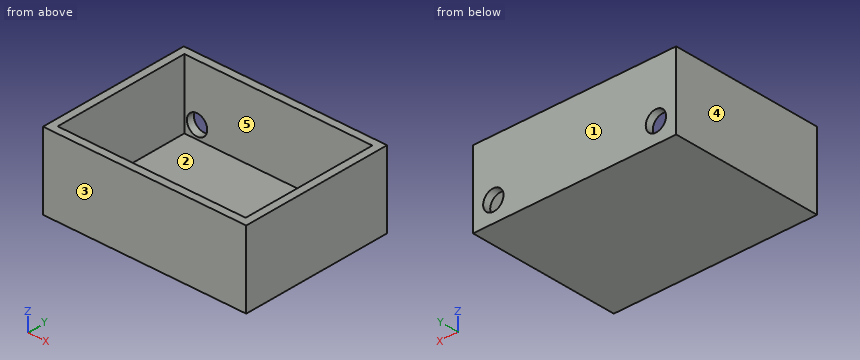
from build123d import *

# Parameters (mm, degrees)
F0_W     = 74
F0_H     = 54
F1_DEPTH = 3
F0_W_2   = 80
F0_H_2   = 60
F2_DEPTH = 30
F3_R     = 4
F4_DEPTH = 5


with BuildPart() as f1:
    # F0 (on Top) → F1 (new body)
    with BuildSketch(Plane.XY):
        with Locations((40, -30)):
            Rectangle(F0_W, F0_H)
    extrude(amount=F1_DEPTH)

    # F0 (on Top) → F2 (join)
    with BuildSketch(Plane.XY):
        with Locations((40, -30)):
            Rectangle(F0_W_2, F0_H_2)
        with Locations((40, -30)):
            Rectangle(F0_W, F0_H, mode=Mode.SUBTRACT)
    extrude(amount=F2_DEPTH)

    # F3 (on Front) → F4 (cut)
    with BuildSketch(Plane.XZ):
        with Locations((72, 8)):
            Circle(F3_R)
        with Locations((8, 8)):
            Circle(F3_R)
    extrude(amount=F4_DEPTH, mode=Mode.SUBTRACT)


solid = f1.part
Check sheet for the modelled part. Datum: model origin and axes. Units: mm. Face numbers are marked on the shaded views. A direction names the side the tool comes from. Give positions to 0.01 mm unless a question says otherwise; leave off trailing zeros. Write each loop counter-clockwise with the first axis right and the second up, starting at its lowest first coordinate (ties: lowest second). Pieces come first, ordered by that corner, then holes. Notation, with made-up numbers: (15, 10) -> (30, 10) arc R32 ccw to (30, 45) -> close; hole circle Ø7 at (-14, -9). An arc over 180 degrees is marked (long way). Use one line per item in the form item = value. Start each with the question number.
1. Section check B-B (x = 8). Record the cut outline in (y, z), and give its area (3 significant figures).
2. Section check D-D (x = 66.5). Record the cut outline in (y, z).
3. Access from +Z, -Z, +X, -X, +Y, -Y to the whole of each face (thin tool, end or side, straight path). Record for the marked faces 4 and 5.
4. Go/stop test with a flat-tipped pin: P1, Ø5, axis at x = 24, y = -22, coming from the +Z side. Record where the tip stops, or that it passes through.
5. Section check A-A (z = 9.75). Record the cut outline in (x, y), and give its area (3 significant figures).
6. Section check C-C (y = -41). Record the cut outline in (x, z).
7. Mould release check, pull along Y, two halves, no side actions. Record for the marked faces 1, 2 and 3: pulls with the +Y half, pulls with the -Y half, needs draft (parallel to the pull), parting line crosses it, or undercut.
8. Thickness scan on line 1 along X through (y, z) = (-1.8, 8); line 2 along X through (y, z) = (-35.5, 8.25); line 3 along Y through (x, z) = (64.5, 12.5). Record the ranges inside material, lowest first. Write a range as from..to.
Conclusion:
q1.outline = (-60, 0) -> (0, 0) -> (0, 4) -> (-3, 4) -> (-3, 3) -> (-57, 3) -> (-57, 30) -> (-60, 30) -> close; (-3, 12) -> (0, 12) -> (0, 30) -> (-3, 30) -> close
q1.area = 318 mm²
q2.outline = (-60, 0) -> (0, 0) -> (0, 30) -> (-3, 30) -> (-3, 3) -> (-57, 3) -> (-57, 30) -> (-60, 30) -> close
q3.face_4 = +Z, -Z, -X, +Y, -Y
q3.face_5 = +Z
q4.P1 = 3
q5.outline = (0, -60) -> (80, -60) -> (80, 0) -> (75.6, 0) -> (75.6, -3) -> (77, -3) -> (77, -57) -> (3, -57) -> (3, -3) -> (4.4, -3) -> (4.4, 0) -> (0, 0) -> close; (11.6, -3) -> (68.4, -3) -> (68.4, 0) -> (11.6, 0) -> close
q5.area = 761 mm²
q6.outline = (0, 0) -> (80, 0) -> (80, 30) -> (77, 30) -> (77, 3) -> (3, 3) -> (3, 30) -> (0, 30) -> close
q7.face_1 = pulls with the +Y half
q7.face_2 = undercut
q7.face_3 = pulls with the -Y half
q8.line_1 = 0..4, 12..68, 76..80
q8.line_2 = 0..3, 77..80
q8.line_3 = -60..-57, -3..0
